from build123d import *

# Parameters (mm, degrees)
SKETCH1_R               = 15.7
SKETCH1_R_2             = 3.3
SKETCH1_R_3             = 2.2
BOSS_EXTRUDE1_DEPTH     = 1.5
SKETCH2_W               = 12.2
SKETCH2_H               = 4.4
BOSS_EXTRUDE2_DEPTH     = 65
CUT_EXTRUDE1_DEPTH      = 71.633915366
CUT_EXTRUDE1_DEPTH_BACK = 90


with BuildPart() as part:
    # Sketch1 → Boss-Extrude1 (new body)
    with BuildSketch(Plane(origin=(0, 0, 0), x_dir=(1, 0, 0), z_dir=(0, 1, 0))):
        with Locations(Location((0, 0, 0), (0, 0, 270))):
            Circle(SKETCH1_R)
        with Locations(Location((0, 0, 0), (0, 0, 270))):
            Circle(SKETCH1_R_2, mode=Mode.SUBTRACT)
        with Locations(Location((-8.3, 0, 0), (0, 0, 270))):
            Circle(SKETCH1_R_3, mode=Mode.SUBTRACT)
        with Locations(Location((8.3, 0, 0), (0, 0, 270))):
            Circle(SKETCH1_R_3, mode=Mode.SUBTRACT)
    extrude(amount=BOSS_EXTRUDE1_DEPTH)

    # Sketch2 → Boss-Extrude2 (add)
    with BuildSketch(Plane(origin=(0, 1.5, 0), x_dir=(1, 0, 0), z_dir=(0, 1, 0))):
        Rectangle(SKETCH2_W, SKETCH2_H)
    extrude(amount=BOSS_EXTRUDE2_DEPTH)

    # Sketch4 → Cut-Extrude1 (cut, two sides: drawn at the far end of the back side and taken through both)
    with BuildSketch(Plane.XY.offset(2.2).offset(-CUT_EXTRUDE1_DEPTH_BACK)):
        with BuildLine():
            ThreePointArc((3.3, 11.5), (2.333452378, 13.833452378), (0, 14.8))
            Line((0, 14.8), (0, 1.5))
            Line((0, 1.5), (2.459674775, 1.5))
            Line((2.459674775, 1.5), (3.3, 1.5))
            Line((3.3, 1.5), (3.3, 11.5))
        make_face()
        with BuildLine():
            Line((-3.3, 11.5), (-3.3, 1.5))
            Line((-3.3, 1.5), (-2.459674775, 1.5))
            Line((-2.459674775, 1.5), (0, 1.5))
            Line((0, 1.5), (0, 14.8))
            ThreePointArc((0, 14.8), (-2.333452378, 13.833452378), (-3.3, 11.5))
        make_face()
    extrude(amount=CUT_EXTRUDE1_DEPTH + CUT_EXTRUDE1_DEPTH_BACK, mode=Mode.SUBTRACT)


solid = part.part
Here's how the part is built. I have some questions about the finished solid (model axes, mm). A direction names the side the tool comes from. Coordinates: 2 decimals unless noted, no trailing zeros. Write each loop counter-clockwise with the first axis right and the second up, starting at its lowest first coordinate (ties: lowest second). Pieces come first, ordered by that corner, then holes.
Item 1: If we mould it in two halves opening along Y, with no side actions, what happens to faces 5 (the flat face through (-3.3, 7, 0)), 6 (the flat face through (4, 0, 0)), 7 (the flat face through (0, 34, 2.2))? For each: +Y half, -Y half, draft (parallel to the pull), parting line (faces both ways), or undercut.
Item 2: On a 3-axis mill with a long thin cutter (end or side, diameter ignored), from which of +Z, -Z, +X, -X, +Y, -Y can I reach the whole of each face in a straight line? I mean faces 1 (the flat face through (3.3, 6, 0)), 2 (the flat face through (0, 34, -2.2)), 3 (the cylindrical face through (-2.008, 0.74, -2.619)), 4 (the flat face through (-6.1, 34, 0)). Say none if no direction works.
Item 3: Will these pins go through, and if not, where does the flat tip stop? pin 1 (10 mm diameter, centred on x = 0.5, y = 45, fed in from +Z); pin 2 (5 mm diameter, centred on y = 42, z = -1, fed in from -X); pin 3 (5 mm diameter, centred on x = -12, z = -0.5, fed in from +Y).
Item 4: I want a section at B-B on y = 13. Write out the boundary of the cut face in (x, z).
Item 5: If I drill on line 1 (X direction, y = 0.5, z = 0); line 2 (Y direction, x = 2, z = -7); line 3 (X direction, y = 22, z = -2), over which ranges is the centre line in solid material (lowest first)?
Item 6: I want a section at D-D on y = 38. Write out the boundary of the cut face in (x, z), and give its area (3 significant figures).
Item 7: I want a section at C-C on x = -8.3. Write out the boundary of the cut face in (y, z), and give its area (3 significant figures).
Item 8: I want a section at A-A on x = 2. Write out the boundary of the cut face in (y, z), and give its area (3 significant figures).
Findings below:
1. face 5: undercut
1. face 6: -Y half
1. face 7: draft
2. face 1: +Z, -Z
2. face 2: -Z, +X, -X, +Y
2. face 3: -Y
2. face 4: +Z, -Z, -X, +Y
3. pin 1: stops at z = 2.2
3. pin 2: stops at x = -6.1
3. pin 3: stops at y = 1.5
4. outline: (-6.1, -2.2) - (-2.94, -2.2) - (-2.94, 2.2) - (-6.1, 2.2) - close; (2.94, -2.2) - (6.1, -2.2) - (6.1, 2.2) - (2.94, 2.2) - close
5. line 1: x = -15.7 to -10.5, -6.1 to -3.3, 3.3 to 6.1, 10.5 to 15.7
5. line 2: y = 0 to 1.5
5. line 3: x = -6.1 to 6.1
6. outline: (-6.1, -2.2) - (6.1, -2.2) - (6.1, 2.2) - (-6.1, 2.2) - close
6. area: 53.7 mm2
7. outline: (0, -13.33) - (1.5, -13.33) - (1.5, -2.2) - (0, -2.2) - close; (0, 2.2) - (1.5, 2.2) - (1.5, 13.33) - (0, 13.33) - close
7. area: 33.4 mm2
8. outline: (0, -15.57) - (1.5, -15.57) - (1.5, -2.62) - (0, -2.62) - close; (0, 2.62) - (1.5, 2.62) - (1.5, 15.57) - (0, 15.57) - close; (14.12, -2.2) - (66.5, -2.2) - (66.5, 2.2) - (14.12, 2.2) - close
8. area: 269 mm2
